```python
from build123d import *

# Parameters (mm, degrees)
F0_R     = 6.35
F1_DEPTH = 50.8


with BuildPart() as f1:
    # F0 (on Top) → F1 (new body)
    with BuildSketch(Plane.XY):
        with BuildLine():
            ThreePointArc((5.065933, 11.645871), (3.643338, 15.338636), (0, 16.883425))
            ThreePointArc((0, 16.883425), (-3.643338, 15.338636), (-5.065933, 11.645871))
            ThreePointArc((-5.065933, 11.645871), (-6.35, 10.998523), (-7.552654, 10.210163))
            ThreePointArc((-7.552654, 10.210163), (-10.998523, 6.35), (-12.618587, 1.435709))
            ThreePointArc((-12.618587, 1.435709), (-12.7, 0), (-12.618587, -1.435709))
            ThreePointArc((-12.618587, -1.435709), (-15.105317, -4.514095), (-14.621475, -8.441712))
            ThreePointArc((-14.621475, -8.441712), (-11.461979, -10.824541), (-7.552654, -10.210163))
            ThreePointArc((-7.552654, -10.210163), (-6.35, -10.998523), (-5.065933, -11.645871))
            ThreePointArc((-5.065933, -11.645871), (-4.719503, -11.790517), (-4.368949, -11.92486))
            Line((-4.368949, -11.92486), (-4.368949, -9.525))
            Line((-4.368949, -9.525), (-1.193949, -9.525))
            Line((-1.193949, -9.525), (-1.193949, -12.643753))
            ThreePointArc((-1.193949, -12.643753), (1.999251, -12.54165), (5.065933, -11.645871))
            ThreePointArc((5.065933, -11.645871), (6.35, -10.998523), (7.552654, -10.210163))
            ThreePointArc((7.552654, -10.210163), (11.461979, -10.824541), (14.621475, -8.441712))
            ThreePointArc((14.621475, -8.441712), (15.105317, -4.514095), (12.618587, -1.435709))
            ThreePointArc((12.618587, -1.435709), (12.7, 0), (12.618587, 1.435709))
            ThreePointArc((12.618587, 1.435709), (10.998523, 6.35), (7.552654, 10.210163))
            ThreePointArc((7.552654, 10.210163), (6.35, 10.998523), (5.065933, 11.645871))
        make_face()
        with Locations((0, -0.838046)):
            Circle(F0_R, mode=Mode.SUBTRACT)
        with BuildLine():
            ThreePointArc((-12.618587, 1.435709), (-10.998523, 6.35), (-7.552654, 10.210163))
            ThreePointArc((-7.552654, 10.210163), (-11.461979, 10.824541), (-14.621475, 8.441712))
            ThreePointArc((-14.621475, 8.441712), (-15.105317, 4.514095), (-12.618587, 1.435709))
        make_face()
        with BuildLine():
            ThreePointArc((14.621475, 8.441712), (11.461979, 10.824541), (7.552654, 10.210163))
            ThreePointArc((7.552654, 10.210163), (10.998523, 6.35), (12.618587, 1.435709))
            ThreePointArc((12.618587, 1.435709), (15.105317, 4.514095), (14.621475, 8.441712))
        make_face()
        with BuildLine():
            ThreePointArc((-4.368949, -11.92486), (-4.719503, -11.790517), (-5.065933, -11.645871))
            ThreePointArc((-5.065933, -11.645871), (-3.643338, -15.338636), (0, -16.883425))
            ThreePointArc((0, -16.883425), (3.643338, -15.338636), (5.065933, -11.645871))
            ThreePointArc((5.065933, -11.645871), (1.999251, -12.54165), (-1.193949, -12.643753))
            ThreePointArc((-1.193949, -12.643753), (-2.804579, -12.386458), (-4.368949, -11.92486))
        make_face()
    extrude(amount=F1_DEPTH)


solid = f1.part
```
Source: CAD feature listing. Evaluate the final solid. Frame: model axes, mm. A direction names the side the tool comes from. Coordinates: 2 decimals unless noted, no trailing zeros. Loops run counter-clockwise (first coordinate to the right, second up) from the corner with the lowest first, then second, coordinate; pieces in that order, holes last. Notation, with made-up numbers: M 89.5,72.5 L 133.5,72.5 A24 cw 133.5,85.5 Z; hole C 14,-11.5 d2. An arc over 180 degrees is marked long. Use a Markdown table: item, result. Add a question column.
Q1. Section query D-D, the plane y = -2.5. Return loops of the section in (x, z).
Q2. Section query B-B, the plane z = 10. State how many separate pieces and enclosed holes the cut face has, and give its area (3 significant figures).
Q3. First-contact query: pin 1 (10 mm diameter, centred on y = 13, z = 35, fed in from -X); pin 2 (2.5 mm diameter, centred on x = -2, z = 19, fed in from -Y); pin 3 (3.5 mm diameter, centred on y = -11.5, z = 26, fed in from -X). Flat tips, straight axial feed; report the tip coordinate or a pass-through.
Q4. Material intervals for L1, parallel to Y at x = -4, z = 39 (3 decimals); L2, parallel to Y at x = -3.5, z = 11 (3 decimals); L3, parallel to X at y = -4, z = 15, sorted ascending.
Q5. Section query A-A, the plane x = 4. Return loops of the section in (y, z).
Q6. Section query C-C, the plane x = -2.5. Return loops of the section in (y, z) (1 decimal).
Q7. Draft query along Y for faces 5 (the flat face through (7, 0, 50.8)), 6 (the cylindrical face through (-6.33, 11.01, 25.04)), 7 (the flat face through (-3, -9.525, 25)). Return one class per face: pulls with the +Y half, pulls with the -Y half, needs draft (parallel to the pull), parting line crosses it, or undercut.
Q8. Access query for faces 1 (the cylindrical face through (-12.7, 0, 25)), 2 (the flat face through (-1.194, -11, 25)), 3 (the cylindrical face through (6.33, -11.01, 25.04)), 4 (the cylindrical face through (6.367, 10.988, 25.044)). Directions: +Z, -Z, +X, -X, +Y, -Y. A direction counts if a zero-diameter tool reaches every point of the face in a straight line with its end or side. Return the directions, or none.
Result:
| question | item | result |
|---|---|---|
| 1 | outline | M -13.98,0 L -6.13,0 L -6.13,50.8 L -13.98,50.8 Z; M 6.13,0 L 13.98,0 L 13.98,50.8 L 6.13,50.8 Z |
| 2 | separate pieces | 1 |
| 2 | enclosed holes | 2 |
| 2 | area | 580 mm2 |
| 3 | pin 1 | stops at x = -14.85 |
| 3 | pin 2 | stops at y = -16.83 |
| 3 | pin 3 | stops at x = -13.54 |
| 4 | L1 | y = -14.928 to -12.054, -9.525 to -5.77, 4.094 to 14.928 |
| 4 | L2 | y = -15.481 to -12.208, -9.525 to -6.136, 4.46 to 15.481 |
| 4 | L3 | x = -14.93 to -5.51, 5.51 to 14.93 |
| 5 | outline | M -14.93,0 L -5.77,0 L -5.77,50.8 L -14.93,50.8 Z; M 4.09,0 L 14.93,0 L 14.93,50.8 L 4.09,50.8 Z |
| 6 | outline | M -16.2,0 L -12.5,0 L -12.5,50.8 L -16.2,50.8 Z; M -9.5,0 L -6.7,0 L -6.7,50.8 L -9.5,50.8 Z; M 5,0 L 16.2,0 L 16.2,50.8 L 5,50.8 Z |
| 7 | face 5 | needs draft |
| 7 | face 6 | pulls with the +Y half |
| 7 | face 7 | undercut |
| 8 | face 1 | +Z, -Z, -X |
| 8 | face 2 | +Z, -Z |
| 8 | face 3 | +Z, -Z, -Y |
| 8 | face 4 | +Z, -Z, +Y |
